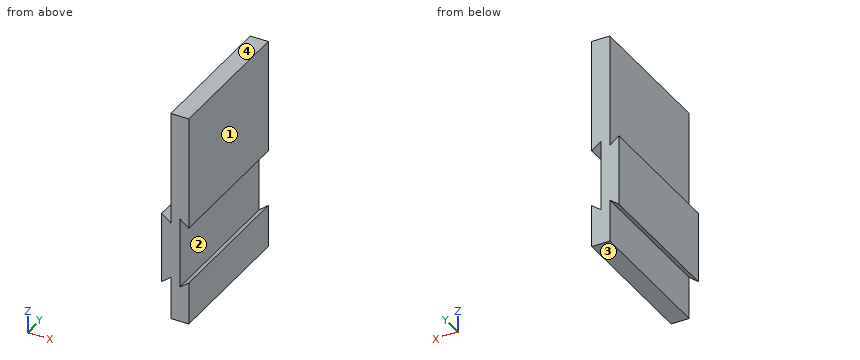
```python
from build123d import *

# Parameters (mm, degrees)
BOSS_EXTRUDE1_DEPTH = 20


with BuildPart() as part:
    # Sketch1 → Boss-Extrude1 (new body)
    with BuildSketch(Plane(origin=(0, 0, 0), x_dir=(1, 0, 0), z_dir=(0, 1, 0))):
        Polygon((0, 5), (1.27, 4), (1.27, 10), (-1.27, 10), (-1.27, 4), (-1.27, -4), (-1.27, -20), (1.27, -20), (1.27, -5), (1.27, -4), (0, -5), align=None)
        Polygon((-2.54, 5), (-2.54, -5), (-1.27, -4), (-1.27, 4), align=None)
    extrude(amount=BOSS_EXTRUDE1_DEPTH)


solid = part.part
```
Can you work these out from the model? Positions are in its coordinate system, mm. Face numbers are marked on the shaded views. Coordinates: 2 decimals unless noted, no trailing zeros. Order: outer loops, then holes, each group sorted by start corner. A loop starts at its lowest first (then second) coordinate and runs counter-clockwise, first axis right, second up.
1. If we section it at A-A (y = 14.25): Please give me the cut outline in (x, z).
2. If we section it at C-C (z = 9.75): Please give me the cut outline in (x, y), then the cut area to 3 significant figures.
3. If we section it at D-D (x = -2.1): Please give me the cut outline in (y, z).
4. I'm going to push flat-ended pins straight in: pin 1 (1.5 mm diameter, centred on y = 11.5, z = 1, fed in from +X); pin 2 (5 mm diameter, centred on y = 11, z = 10.5, fed in from -X). Where does each tip first touch, or does it pass through?
5. Thinking about a two-plate mould opening in Z: for the marked faces 1, 2, 3 and 4, which applies, +Z half, -Z half, draft (parallel to the pull), parting line (faces both ways), or undercut?
6. I need wall thicknesses on line 1 (X direction, y = 17.25, z = 6.75); line 2 (X direction, y = 8.5, z = 1.75); line 3 (Z direction, x = 0.25, y = 11.25). Which ranges of each line are inside material? Lowest first, please.
7. If we section it at B-B (x = 0.9): Please give me the cut outline in (y, z), then the cut area to 3 significant figures.
Entries:
1. outline: (-2.54, -5) - (-1.27, -4) - (-1.27, -10) - (1.27, -10) - (1.27, -4) - (0, -5) - (0, 5) - (1.27, 4) - (1.27, 20) - (-1.27, 20) - (-1.27, 4) - (-2.54, 5) - close
2. outline: (-1.27, 0) - (1.27, 0) - (1.27, 20) - (-1.27, 20) - close
2. area: 50.8 mm2
3. outline: (0, -4.65) - (20, -4.65) - (20, 4.65) - (0, 4.65) - close
4. pin 1: stops at x = 0
4. pin 2: stops at x = -1.27
5. face 1: draft
5. face 2: undercut
5. face 3: -Z half
5. face 4: +Z half
6. line 1: x = -1.27 to 1.27
6. line 2: x = -2.54 to 0
6. line 3: z = -10 to -4.8, 4.8 to 20
7. outline: (0, -10) - (20, -10) - (20, -4.29) - (0, -4.29) - close; (0, 4.29) - (20, 4.29) - (20, 20) - (0, 20) - close
7. area: 428 mm2
